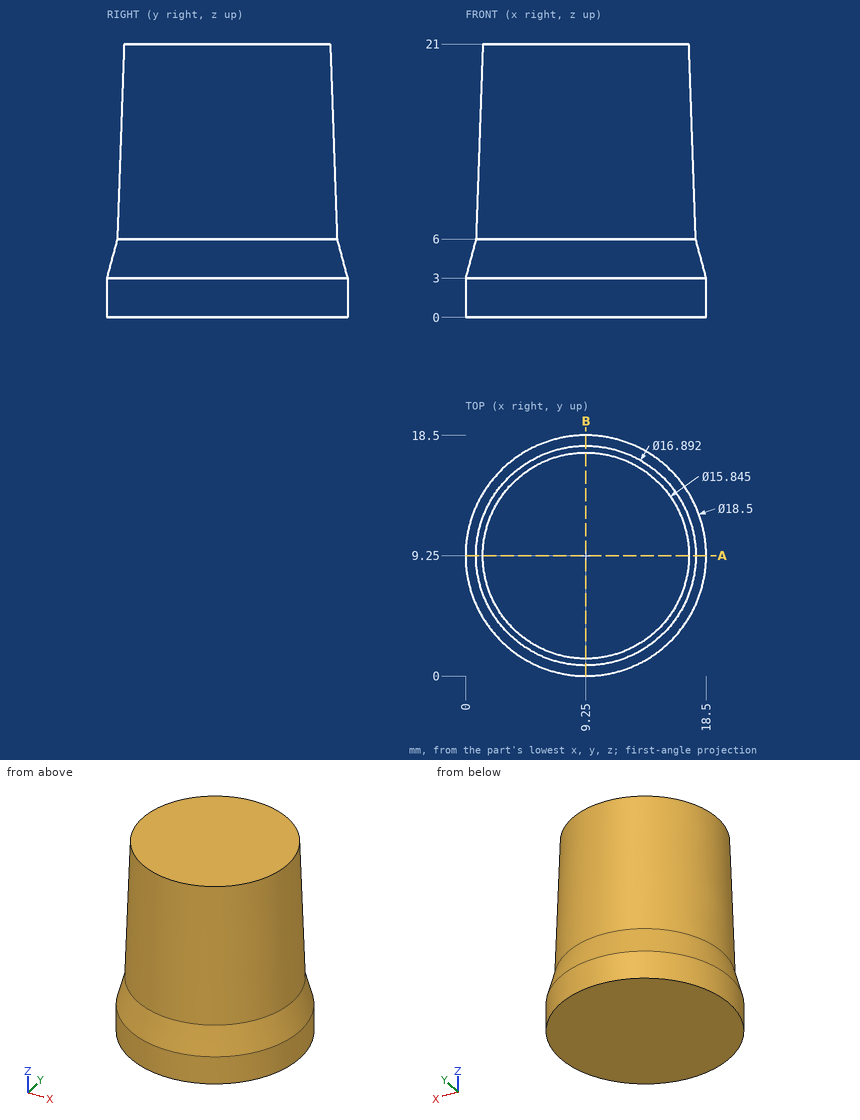
The drawing under review shows one solid part. Ordinate dimensions are in mm from its lowest x, y, z. Give positions to 0.01 mm unless a question says otherwise; leave off trailing zeros. Order: outer loops, then holes, each group sorted by start corner. A loop starts at its lowest first (then second) coordinate and runs counter-clockwise, first axis right, second up. Notation, with made-up numbers: (45.5, -27.5) -> (93.5, -27.5) arc R13 cw to (93.5, -5.5) -> close; hole circle Ø4 at (10.25, 37). An arc over 180 degrees is marked (long way). Write item = value, one per line.
1) Insertion check: pin 1 (1 mm diameter, centred on x = 4.5, z = 11, fed in from -Y); pin 2 (3 mm diameter, centred on y = 4.5, z = 8, fed in from -X); pin 3 (2 mm diameter, centred on y = 4, z = 10.5, fed in from +X). Each pin has a flat end and moves straight along its axis. Give the tip position at first contact, or say it passes through.
Findings:
pin_1 = 2.15
pin_2 = 1.53
pin_3 = 16.37
2) To check wall thickness, follow L1, parallel to X at y = 3.25, z = 12; L2, parallel to Y at x = 17.75, z = 2.75; L3, parallel to Y at x = 6.25, z = 6.25 (1 decimal). State the ranges of each line that lie inside material, in increasing order. Write a range as from..to.
Findings:
L1 = 3.61..14.89
L2 = 5.6..12.9
L3 = 1.4..17.1
3) We need section A-A, the plane y = 9.25. Give the boundary of the cut face in (x, z).
Findings:
outline = (0, 0) -> (18.5, 0) -> (18.5, 3) -> (17.7, 6) -> (17.17, 21) -> (1.33, 21) -> (0.8, 6) -> (0, 3) -> close
